Input: part model. Units: mm. Frame: model coordinates. Face numbers are marked on the shaded views. A direction names the side the tool comes from. Give positions to 0.01 mm unless a question says otherwise; leave off trailing zeros. Write each loop counter-clockwise with the first axis right and the second up, starting at its lowest first coordinate (ties: lowest second). Pieces come first, ordered by that corner, then holes. Notation, with made-up numbers: (54, 49) -> (85, 49) arc R13 ccw to (85, 55) -> close; hole circle Ø4 at (17.5, 42.5). An arc over 180 degrees is marked (long way). Return JSON: item names as keys, results as strings. Group by question number.
Item 1: Section D-D, the plane y = -1.5. Return loops of the section in (x, z), then the cut area to 3 significant figures.
Item 2: Mould query, pull axis X, two halves, no side actions, for the marked faces 1, 2 and 3. Classes: released by +X, released by -X, zero draft, split by the parting line, or undercut.
Item 3: Section C-C, the plane x = -1.25. Count the separate pieces of the cut face and the enclosed holes in it, then the cut area to 3 significant figures.
Item 4: Set-up query: the marked faces 4 and 5. Return all of +Z, -Z, +X, -X, +Y, -Y with unobstructed straight access to the full face (end or side cutting, diameter ignored); none if empty.
Item 5: Section A-A, the plane y = -5.5. Return loops of the section in (x, z), then the cut area to 3 significant figures.
Item 6: Section B-B, the plane y = -3. Return loops of the section in (x, z), then the cut area to 3 significant figures.
Item 7: Line query: line 1 (Z direction, x = 4.25, y = -4.5); line 2 (Z direction, x = 5.75, y = 2.5); line 3 (Y direction, x = -2.5, z = 3). Output: solid intervals per line, ascending. Write a range as [from, to].
Item 8: Pin query (flat end, axial travel): P1, Ø2, axis at x = 6.5, y = 3, coming from the +Z side; P2, Ø4, axis at x = -8.5, y = -2, coming from the -Z side; P3, Ø6, axis at x = 1, y = 2, coming from the +Z side. Return the tip coordinate at first contact, or that it passes through.
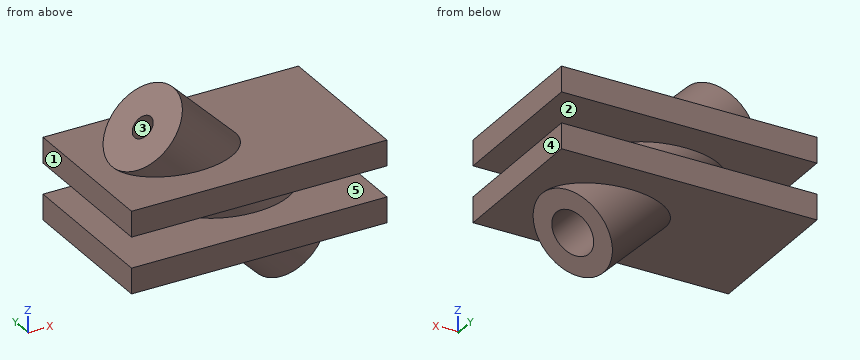
from build123d import *

# Parameters (mm, degrees)
SKETCH001_W = 4.25
SKETCH001_H = 20
SKETCH002_W = 25
SKETCH002_H = 2.5
PAD_DEPTH   = 7.5


with BuildPart() as part:
    # Sketch001 → Revolution (revolve)
    with BuildSketch(Plane(origin=(0, 0, 0), x_dir=(0.707107, 0, 0.707107), z_dir=(0, -1, 0))):
        with Locations((2.125, 0)):
            Rectangle(SKETCH001_W, SKETCH001_H)
    revolve(axis=Axis((0, 0, 0), (-0.707107, 0, 0.707107)))

    # Sketch002 → Pad (new body, symmetric)
    with BuildSketch(Plane.XZ):
        with Locations((0, 2.75)):
            Rectangle(SKETCH002_W, SKETCH002_H)
    pad = extrude(amount=PAD_DEPTH, both=True)

    # Mirrored: Pad across Sketch002 H_Axis
    add(pad.mirror(Plane(origin=(0, 0, 0), x_dir=(0, -1, 0), z_dir=(0, 0, 1))))

    # Sketch → Groove (revolve, cut)
    with BuildSketch(Plane(origin=(0, 0, 0), x_dir=(0.707107, 0, 0.707107), z_dir=(0, -1, 0))):
        Polygon((0, -10), (2.25, -10), (2.25, 0), (1.125, 0), (1.125, 10), (0, 10), align=None)
    revolve(axis=Axis((0, 0, 0), (-0.707107, 0, 0.707107)), mode=Mode.SUBTRACT)


solid = part.part
Answer below:
{
 "1": {"outline": "(-12.5, -4) -> (-1.62, -4) -> (4.26, -9.88) -> (5.89, -8.26) -> (-1.19, -1.19) -> (1.19, 1.19) -> (8.26, -5.89) -> (9.88, -4.26) -> (9.62, -4) -> (12.5, -4) -> (12.5, -1.5) -> (7.12, -1.5) -> (4.12, 1.5) -> (12.5, 1.5) -> (12.5, 4) -> (1.62, 4) -> (-4.26, 9.88) -> (-9.88, 4.26) -> (-9.62, 4) -> (-12.5, 4) -> (-12.5, 1.5) -> (-7.12, 1.5) -> (-4.12, -1.5) -> (-12.5, -1.5) -> close", "area": "194 mm2"},
 "2": {"face 1": "released by -X", "face 2": "zero draft", "face 3": "undercut"},
 "3": {"separate pieces": "1", "enclosed holes": "2", "area": "112 mm2"},
 "4": {"face 4": "+Z, -Z, +X, +Y, -Y", "face 5": "none"},
 "5": {"outline": "(-12.5, -4) -> (12.5, -4) -> (12.5, -1.5) -> (-12.5, -1.5) -> close; (-12.5, 1.5) -> (12.5, 1.5) -> (12.5, 4) -> (-12.5, 4) -> close", "area": "125 mm2"},
 "6": {"outline": "(-12.5, -4) -> (-0.26, -4) -> (4.94, -9.2) -> (9.2, -4.94) -> (8.26, -4) -> (12.5, -4) -> (12.5, -1.5) -> (5.76, -1.5) -> (2.76, 1.5) -> (12.5, 1.5) -> (12.5, 4) -> (0.26, 4) -> (-4.94, 9.2) -> (-9.2, 4.94) -> (-8.26, 4) -> (-12.5, 4) -> (-12.5, 1.5) -> (-5.76, 1.5) -> (-2.76, -1.5) -> (-12.5, -1.5) -> close", "area": "203 mm2"},
 "7": {"line 1": "z = [-4, -1.5], [1.5, 4]", "line 2": "z = [-8.39, -0.89], [1.5, 4]", "line 3": "y = [-7.5, -1.07], [1.07, 7.5]"},
 "8": {"P1": "stops at z = 4", "P2": "stops at z = -4", "P3": "stops at z = 7.67"}
}
